The listing builds one solid part. Answer for the finished solid, in the listing's coordinates (mm). A direction names the side the tool comes from. Coordinates: 2 decimals unless noted, no trailing zeros. Loops run counter-clockwise (first coordinate to the right, second up) from the corner with the lowest first, then second, coordinate; pieces in that order, holes last. Notation, with made-up numbers: M 53.5,33.5 L 64.5,33.5 A28 cw 64.5,51.5 Z; hole C -1.75,8 d2. An arc over 180 degrees is marked long. Return JSON: item names as keys, results as strings. Group by question number.
1. Section A-A (z = 6.3) is taken. Write down the section's boundary in (x, y), then the cut area to 3 significant figures.
2. Section C-C (z = -1.5) is taken. Write down the section's boundary in (x, y).
3. Which of the six approach directions +Z, -Z, +X, -X, +Y, -Y give full straight-line access (tool end or side, diameter ignored) to faces 1 (the face through (24, 26, 0)), 2 (the face through (-24, 26, 0)), 3 (the face through (-24, 28.5, 0)), 4 (the face through (24, 28.5, 0))?
4. The mould has two halves that part along X. Classify faces 5 (the face through (26.198, 27.232, -6.388)), 6 (the face through (-27.5, 27, 0)), 7 (the face through (-26.047, 27.232, -5.534)), 8 (the face through (0, 18, 10)): pulls with the +X half, pulls with the -X half, needs draft (parallel to the pull), parting line crosses it, or undercut.
5. Given P1, Ø1.5, axis at x = -10, z = 2, coming from the +Y side; P2, Ø6.5, axis at x = -24.2, z = 6.3, coming from the -Y side; P3, Ø4, axis at x = 25, z = -4.5, coming from the +Y side; P4, Ø2, axis at x = 9.625, z = 0.275, coming from the +Y side, each flat-ended and moving along its own axis, determine where each tip first touches the part or whether it passes through.
6. Straight lines are drawn through the part: L1, parallel to Z at x = 24.2, y = 27.8; L2, parallel to Y at x = 6, z = 6.25; L3, parallel to X at y = 6.5, z = 3.75. For each, find the intervals that lie inside material, in ascending order. Write a range as from..to.
7. Section B-B (x = -24.2) is taken. Write down the section's boundary in (y, z).
8. Section D-D (x = 23.5) is taken. Write down the section's boundary in (y, z), then the cut area to 3 significant figures.
```python
from build123d import *

# Parameters (mm, degrees)
SKETCH1_W                        = 40
SKETCH1_H                        = 20
BOSS_EXTRUDE1_DEPTH              = 37
SKETCH2_W                        = 7.5
SKETCH2_H                        = 20
BOSS_EXTRUDE2_DEPTH              = 2.5
F_4_0_4_DIAMETER_HOLE1_D         = 4
SKETCH5_R                        = 2.875
BOSS_EXTRUDE3_DEPTH              = 4
F_1_85_1_85_DIAMETER_HOLE1_D     = 1.85
F_1_85_1_85_DIAMETER_HOLE1_DEPTH = 4
F_1_85_1_85_DIAMETER_HOLE1_TIP   = 0.555796073


with BuildPart() as part:
    # Sketch1 → Boss-Extrude1 (new body)
    with BuildSketch(Plane(origin=(0, 0, 0), x_dir=(1, 0, 0), z_dir=(0, 1, 0))):
        Rectangle(SKETCH1_W, SKETCH1_H)
    extrude(amount=BOSS_EXTRUDE1_DEPTH)

    # Sketch2 → Boss-Extrude2 (add)
    with BuildSketch(Plane(origin=(0, 26, 0), x_dir=(1, 0, 0), z_dir=(0, 1, 0))):
        with Locations((23.75, 0)):
            Rectangle(SKETCH2_W, SKETCH2_H)
        with Locations((-23.75, 0)):
            Rectangle(SKETCH2_W, SKETCH2_H)
    extrude(amount=BOSS_EXTRUDE2_DEPTH)

    # Ø4.0 (4) Diameter Hole1 (through all)
    with Locations(Plane(origin=(0, 28.5, 0), x_dir=(1, 0, 0), z_dir=(0, 1, 0))):
        with Locations((-24.2, -6.3), (-24.2, 6.3), (24.2, 6.3), (24.2, -6.3)):
            Hole(F_4_0_4_DIAMETER_HOLE1_D / 2)

    # Sketch5 → Boss-Extrude3 (add)
    with BuildSketch(Plane(origin=(0, 37, 0), x_dir=(1, 0, 0), z_dir=(0, 1, 0))):
        with Locations(Location((9.625, -0.275, 0), (0, 0, 90))):
            Circle(SKETCH5_R)
    extrude(amount=BOSS_EXTRUDE3_DEPTH)

    # Ø1.85 (1.85) Diameter Hole1
    with Locations(Plane(origin=(0, 41, 0), x_dir=(1, 0, 0), z_dir=(0, 1, 0))):
        with Locations((9.625, -0.275)):
            Hole(F_1_85_1_85_DIAMETER_HOLE1_D / 2, depth=F_1_85_1_85_DIAMETER_HOLE1_DEPTH)
            with Locations((0, 0, -(F_1_85_1_85_DIAMETER_HOLE1_DEPTH + F_1_85_1_85_DIAMETER_HOLE1_TIP / 2))):  # 118° drill point
                Cone(0, F_1_85_1_85_DIAMETER_HOLE1_D / 2, F_1_85_1_85_DIAMETER_HOLE1_TIP, mode=Mode.SUBTRACT)


solid = part.part
```
Worked out:
{
 "1": {"outline": "M -27.5,26 L -26.2,26 L -26.2,28.5 L -27.5,28.5 Z; M -22.2,26 L -20,26 L -20,0 L 20,0 L 20,26 L 22.2,26 L 22.2,28.5 L 20,28.5 L 20,37 L -20,37 L -20,28.5 L -22.2,28.5 Z; M 26.2,26 L 27.5,26 L 27.5,28.5 L 26.2,28.5 Z", "area": "1,500 mm^2"},
 "2": {"outline": "M -27.5,26 L -20,26 L -20,0 L 20,0 L 20,26 L 27.5,26 L 27.5,28.5 L 20,28.5 L 20,37 L 11.89,37 L 11.89,41 L 7.36,41 L 7.36,37 L -20,37 L -20,28.5 L -27.5,28.5 Z"},
 "3": {"face 1": "+Z, -Z, +X, -Y", "face 2": "+Z, -Z, -X, -Y", "face 3": "+Z, -Z, -X, +Y", "face 4": "+Z, -Z, +X, +Y"},
 "4": {"face 5": "undercut", "face 6": "pulls with the -X half", "face 7": "undercut", "face 8": "needs draft"},
 "5": {"P1": "y = 37", "P2": "y = 26", "P3": "y = 28.5", "P4": "y = 41"},
 "6": {"L1": "-10..-8.3, -4.3..4.3, 8.3..10", "L2": "0..37", "L3": "-20..20"},
 "7": {"outline": "M 26,-10 L 28.5,-10 L 28.5,-8.3 L 26,-8.3 Z; M 26,-4.3 L 28.5,-4.3 L 28.5,4.3 L 26,4.3 Z; M 26,8.3 L 28.5,8.3 L 28.5,10 L 26,10 Z"},
 "8": {"outline": "M 26,-10 L 28.5,-10 L 28.5,-8.17 L 26,-8.17 Z; M 26,-4.43 L 28.5,-4.43 L 28.5,4.43 L 26,4.43 Z; M 26,8.17 L 28.5,8.17 L 28.5,10 L 26,10 Z", "area": "31.3 mm^2"}
}
